Here's how the part is built. I have some questions about the finished solid (model axes, mm). A direction names the side the tool comes from. Coordinates: 2 decimals unless noted, no trailing zeros. Write each loop counter-clockwise with the first axis right and the second up, starting at its lowest first coordinate (ties: lowest second). Pieces come first, ordered by that corner, then holes.
Item 1: I'm going to push flat-ended pins straight in: pin 1 Ø14 at (x, y) = (13.5, 13.5) entering from +Z; pin 2 Ø1.2 at (x, y) = (2.96, 2.96) entering from +Z. Where does each tip first touch, or does it pass through?
Item 2: If we section it at A-A (z = 6): Please give me the cut outline in (x, y) (3 decimals).
Item 3: We'd pull the mould along X, two halves only. Please class faces 3 (the face through (3, 21, 23.178)), 4 (the face through (15, 12, 4.191)), 5 (the face through (0, 14, 14)), 6 (the face through (19, 0, 14)): +X half, -X half, draft (parallel to the pull), parting line (faces both ways), or undercut.
Item 4: If we section it at B-B (x = 8): Please give me the cut outline in (y, z) (3 decimals).
Item 5: If we section it at C-C (y = 9.5): Please give me the cut outline in (x, z) (3 decimals), then the cut area to 3 significant figures.
Item 6: For faces 1 (the face through (18, 15, 0)), 2 (the face through (34, 3, 23.178)), which set-ups out of +Z, -Z, +X, -X, +Y, -Y let a thin tool reach every point of the face, with its end or its side?
Item 7: If I drill on line 1 (X direction, y = 10, z = 3) (3 decimals); line 2 (Y direction, x = 27, z = 1.5); line 3 (X direction, y = 8, z = 6) (3 decimals), over which ranges is the centre line in solid material (lowest first)?
Item 8: If we section it at D-D (z = 24): Please give me the cut outline in (x, y) (3 decimals).
from build123d import *

# Parameters (mm, degrees)
SKETCH2_W           = 37.465
SKETCH2_H           = 24.13
BOSS_EXTRUDE1_DEPTH = 24.892
CUT_EXTRUDE1_DEPTH  = 20.701
CUT_EXTRUDE3_DEPTH  = 4.191
FILLET1_R           = 5.08
BOSS_EXTRUDE3_START = 2.286
BOSS_EXTRUDE3_DEPTH = 2.286
SKETCH8_R           = 1.905
CUT_EXTRUDE4_DEPTH  = 7.62
BOSS_EXTRUDE5_START = 2.286
BOSS_EXTRUDE5_DEPTH = 2.286
SKETCH10_R          = 1
CUT_EXTRUDE5_DEPTH  = 4


with BuildPart() as part:
    # Sketch2 → Boss-Extrude1 (new body)
    with BuildSketch(Plane.XY):
        with Locations((18.7325, 12.065)):
            Rectangle(SKETCH2_W, SKETCH2_H)
    extrude(amount=BOSS_EXTRUDE1_DEPTH)

    # Sketch3 → Cut-Extrude1 (cut)
    with BuildSketch(Plane.XY.offset(24.892)):
        with BuildLine():
            ThreePointArc((3.175, 16.637), (4.439712919, 19.690287081), (7.493, 20.955))
            Line((7.493, 20.955), (29.972, 20.955))
            ThreePointArc((29.972, 20.955), (33.025287081, 19.690287081), (34.29, 16.637))
            Line((34.29, 16.637), (34.29, 7.493))
            ThreePointArc((34.29, 7.493), (33.025287081, 4.439712919), (29.972, 3.175))
            Line((29.972, 3.175), (7.493, 3.175))
            ThreePointArc((7.493, 3.175), (4.439712919, 4.439712919), (3.175, 7.493))
            Line((3.175, 7.493), (3.175, 16.637))
        make_face()
    extrude(amount=-CUT_EXTRUDE1_DEPTH, mode=Mode.SUBTRACT)

    # Sketch4 → Cut-Extrude3 (cut)
    with BuildSketch(Plane.XY.offset(4.191)):
        with BuildLine():
            Line((32.086974483, 8.570131), (32.07077796, 10.882539488))
            add(Edge.make_bspline(
                [(32.07077796, 10.882539488), (32.073215089, 11.03512727), (32.05346317, 11.384531492), (31.98348624, 11.89897185), (31.690265244, 12.891461502), (30.781603575, 14.240804474), (29.41900903, 15.119220909), (28.414706523, 15.393168176), (27.909381539, 15.452204781), (27.554769457, 15.464756938), (27.429691001, 15.46229384)],
                knots=[0, 0, 0, 0.046875, 0.09375, 0.1875, 0.375, 0.625, 0.8125, 0.90625, 0.953125, 1, 1, 1], degree=2))
            Line((27.429691001, 15.46229384), (21.587714207, 15.44582783))
            add(Edge.make_bspline(
                [(21.587714207, 15.44582783), (21.462803996, 15.448731855), (21.106730304, 15.437338634), (20.595765352, 15.378996632), (19.591692577, 15.107051395), (18.225687665, 14.229774678), (17.316214622, 12.885953496), (17.020022679, 11.889285009), (16.949885556, 11.382167163), (16.92906595, 11.034797324), (16.930958193, 10.882006896)],
                knots=[0, 0, 0, 0.046875, 0.09375, 0.1875, 0.375, 0.625, 0.8125, 0.90625, 0.953125, 1, 1, 1], degree=2))
            Line((16.930958193, 10.882006896), (16.947147256, 8.570663591))
            add(Edge.make_bspline(
                [(16.947147256, 8.570663591), (16.944692803, 8.418076087), (16.96440505, 8.068669624), (17.034323571, 7.554221325), (17.32743188, 6.561698387), (18.235940341, 5.212252256), (19.598435143, 4.33368112), (20.60270654, 4.059619828), (21.108024818, 4.00052585), (21.462635472, 3.98793343), (21.587714207, 3.990382327)],
                knots=[0, 0, 0, 0.046875, 0.09375, 0.1875, 0.375, 0.625, 0.8125, 0.90625, 0.953125, 1, 1, 1], degree=2))
            Line((21.587714207, 3.990382327), (27.429691002, 4.006848338))
            add(Edge.make_bspline(
                [(27.429691002, 4.006848338), (27.554600877, 4.003929875), (27.910675883, 4.015281941), (28.421647575, 4.073564883), (29.425751775, 4.345394065), (30.791858076, 5.22251289), (31.701486436, 6.566228943), (31.997793574, 7.562863188), (32.067989311, 8.069972924), (32.088849066, 8.417340355), (32.086974483, 8.570131)],
                knots=[0, 0, 0, 0.046875, 0.09375, 0.1875, 0.375, 0.625, 0.8125, 0.90625, 0.953125, 1, 1, 1], degree=2))
        make_face()
    extrude(amount=-CUT_EXTRUDE3_DEPTH, mode=Mode.SUBTRACT)

    # Fillet1
    fillet1_edges = [part.edges().sort_by_distance(p)[0] for p in [
        (0, 24.13, 12.446),
        (37.465, 24.13, 12.446),
        (37.465, 0, 12.446),
        (0, 0, 12.446),
    ]]
    fillet(fillet1_edges, radius=FILLET1_R)

    # Sketch7 → Boss-Extrude3 (add)
    with BuildSketch(Plane.XY.offset(24.892).offset(BOSS_EXTRUDE3_START)):
        with BuildLine():
            ThreePointArc((35.59175, 18.3515), (34.252642204, 21.584392204), (31.01975, 22.9235))
            Line((31.01975, 22.9235), (6.44525, 22.9235))
            ThreePointArc((6.44525, 22.9235), (3.212357796, 21.584392204), (1.87325, 18.3515))
            Line((1.87325, 18.3515), (1.87325, 5.7785))
            ThreePointArc((1.87325, 5.7785), (3.212357796, 2.545607796), (6.44525, 1.2065))
            Line((6.44525, 1.2065), (31.01975, 1.2065))
            ThreePointArc((31.01975, 1.2065), (34.252642204, 2.545607796), (35.59175, 5.7785))
            Line((35.59175, 5.7785), (35.59175, 18.3515))
        make_face()
        with BuildLine():
            ThreePointArc((3.175, 16.637), (4.439712919, 19.690287081), (7.493, 20.955))
            Line((7.493, 20.955), (29.972, 20.955))
            ThreePointArc((29.972, 20.955), (33.025287081, 19.690287081), (34.29, 16.637))
            Line((34.29, 16.637), (34.29, 7.493))
            ThreePointArc((34.29, 7.493), (33.025287081, 4.439712919), (29.972, 3.175))
            Line((29.972, 3.175), (7.493, 3.175))
            ThreePointArc((7.493, 3.175), (4.439712919, 4.439712919), (3.175, 7.493))
            Line((3.175, 7.493), (3.175, 16.637))
        make_face(mode=Mode.SUBTRACT)
    extrude(amount=-BOSS_EXTRUDE3_DEPTH)

    # Sketch8 → Cut-Extrude4 (cut)
    with BuildSketch(Plane.ZY):
        with Locations((12.446, 12.065)):
            Circle(SKETCH8_R)
    extrude(amount=-CUT_EXTRUDE4_DEPTH, mode=Mode.SUBTRACT)

    # Sketch9 → Boss-Extrude5 (add)
    with BuildSketch(Plane.XY.offset(24.892).offset(BOSS_EXTRUDE5_START)):
        with BuildLine():
            Line((37.465, 5.08), (37.465, 19.05))
            ThreePointArc((37.465, 19.05), (35.977102448, 22.642102448), (32.385, 24.13))
            Line((32.385, 24.13), (5.08, 24.13))
            ThreePointArc((5.08, 24.13), (1.487897552, 22.642102448), (0, 19.05))
            Line((0, 19.05), (0, 5.08))
            ThreePointArc((0, 5.08), (1.487897552, 1.487897552), (5.08, 0))
            Line((5.08, 0), (32.385, 0))
            ThreePointArc((32.385, 0), (35.977102448, 1.487897552), (37.465, 5.08))
        make_face()
        with BuildLine():
            Line((6.44525, 1.2065), (31.01975, 1.2065))
            ThreePointArc((31.01975, 1.2065), (34.252642204, 2.545607796), (35.59175, 5.7785))
            Line((35.59175, 5.7785), (35.59175, 18.3515))
            ThreePointArc((35.59175, 18.3515), (34.252642204, 21.584392204), (31.01975, 22.9235))
            Line((31.01975, 22.9235), (6.44525, 22.9235))
            ThreePointArc((6.44525, 22.9235), (3.212357796, 21.584392204), (1.87325, 18.3515))
            Line((1.87325, 18.3515), (1.87325, 5.7785))
            ThreePointArc((1.87325, 5.7785), (3.212357796, 2.545607796), (6.44525, 1.2065))
        make_face(mode=Mode.SUBTRACT)
    extrude(amount=-BOSS_EXTRUDE5_DEPTH)

    # Sketch10 → Cut-Extrude5 (cut)
    with BuildSketch(Plane.XY.offset(27.178)):
        with BuildLine():
            ThreePointArc((3.963805235, 21.166194765), (3.346488668, 22.090074297), (2.256698454, 21.873301546))
            Line((2.256698454, 21.873301546), (3.670912016, 20.459087984))
            ThreePointArc((3.670912016, 20.459087984), (3.887684768, 20.783511332), (3.963805235, 21.166194765))
        make_face()
        with BuildLine():
            Line((3.670912016, 20.459087984), (2.256698454, 21.873301546))
            ThreePointArc((2.256698454, 21.873301546), (2.256698454, 20.459087984), (3.670912016, 20.459087984))
        make_face()
        with Locations((34.501194765, 21.166194765)):
            Circle(SKETCH10_R)
        with Locations((34.501194765, 2.963805235)):
            Circle(SKETCH10_R)
        with Locations((2.963805235, 2.963805235)):
            Circle(SKETCH10_R)
    extrude(amount=-CUT_EXTRUDE5_DEPTH, mode=Mode.SUBTRACT)


solid = part.part
Answer list:
1. pin 1: stops at z = 4.19
1. pin 2: stops at z = 23.18
2. outline: (0, 5.08) arc R5.08 ccw to (5.08, 0) - (32.385, 0) arc R5.08 ccw to (37.465, 5.08) - (37.465, 19.05) arc R5.08 ccw to (32.385, 24.13) - (5.08, 24.13) arc R5.08 ccw to (0, 19.05) - close; hole (3.175, 7.493) arc R4.318 ccw to (7.493, 3.175) - (29.972, 3.175) arc R4.318 ccw to (34.29, 7.493) - (34.29, 16.637) arc R4.318 ccw to (29.972, 20.955) - (7.493, 20.955) arc R4.318 ccw to (3.175, 16.637) - close
3. face 3: undercut
3. face 4: undercut
3. face 5: -X half
3. face 6: draft
4. outline: (0, 0) - (24.13, 0) - (24.13, 27.178) - (20.955, 27.178) - (20.955, 4.191) - (3.175, 4.191) - (3.175, 27.178) - (0, 27.178) - close
5. outline: (0, 0) - (16.941, 0) - (16.941, 4.191) - (3.175, 4.191) - (3.175, 27.178) - (0, 27.178) - close; (32.08, 0) - (37.465, 0) - (37.465, 27.178) - (34.29, 27.178) - (34.29, 4.191) - (32.08, 4.191) - close
5. area: 240 mm2
6. face 1: -Z, +X, -X, +Y, -Y
6. face 2: +Z
7. line 1: x = 0 to 16.937, 32.077 to 37.465
7. line 2: y = 0 to 4.01, 15.46 to 24.13
7. line 3: x = 0 to 3.175, 34.29 to 37.465
8. outline: (0, 5.08) arc R5.08 ccw to (5.08, 0) - (32.385, 0) arc R5.08 ccw to (37.465, 5.08) - (37.465, 19.05) arc R5.08 ccw to (32.385, 24.13) - (5.08, 24.13) arc R5.08 ccw to (0, 19.05) - close; hole circle Ø2 at (2.964, 2.964); hole circle Ø2 at (2.964, 21.166); hole (3.175, 7.493) arc R4.318 ccw to (7.493, 3.175) - (29.972, 3.175) arc R4.318 ccw to (34.29, 7.493) - (34.29, 16.637) arc R4.318 ccw to (29.972, 20.955) - (7.493, 20.955) arc R4.318 ccw to (3.175, 16.637) - close; hole circle Ø2 at (34.501, 2.964); hole circle Ø2 at (34.501, 21.166)
